Design review of the part built by this model. Coordinates are the model's own, in mm. Face numbers are marked on the shaded views. A direction names the side the tool comes from. Coordinates: 2 decimals unless noted, no trailing zeros. Loops run counter-clockwise (first coordinate to the right, second up) from the corner with the lowest first, then second, coordinate; pieces in that order, holes last. Notation, with made-up numbers: (38, 13.5) - (79, 13.5) arc R14 cw to (79, 37.5) - close; hole circle Ø10 at (57, -1). An arc over 180 degrees is marked (long way). Use one line per item in the form item = value. Start each with the question number.
(1) Add section D-D (x = -12). State the section outline as (y, z) points, plus the area to 3 significant figures.
(2) For L1, parallel to Y at x = -14.65, z = 0; L2, parallel to X at y = -7.25, z = -5; L3, parallel to Z at x = 39.5, y = -3.75, list the stretches that pass through material, from the lowest coordinate up.
(3) The part is to be moulded in two halves that separate along Z. For the marked faces 1, 2 and 3, say which applies: pulls with the +Z half, pulls with the -Z half, needs draft (parallel to the pull), parting line crosses it, or undercut.
(4) Tool access review of the marked faces 4, 5 and 6: name each direction out of +Z, -Z, +X, -X, +Y, -Y from which nothing blocks a thin tool from reaching the whole face with its end or side.
(5) Clearance check with flat-ended pins moving along their axes: pin 1 Ø3 at (x, y) = (12.5, -6) entering from -Z; pin 2 Ø8 at (x, z) = (37.5, 5.5) entering from +Y; pin 3 Ø1 at (y, z) = (-8, -1.5) entering from -X. State where each tip first meets the part, or that it passes through.
(6) Add section C-C (x = 0). State the section outline as (y, z) points.
(7) Add section A-A (y = 0). State the section outline as (x, z) points.
(8) Add section B-B (x = 24.5). State the section outline as (y, z) points, plus the area to 3 significant figures.
```python
from build123d import *

# Parameters (mm, degrees)
SKETCH_3_W               = 10
SKETCH_3_H               = 2
CUT_EXTRUDE_1_DEPTH      = 46.803930098
PATTERN_CIRCULAR_1_COUNT = 2
PATTERN_CIRCULAR_2_COUNT = 3


with BuildPart() as part:
    # Эскиз1 → Повернуть1 (revolve)
    with BuildSketch(Plane.XY, mode=Mode.PRIVATE) as revolve_1_sk:
        Polygon((-16, 2.55), (-16, 4.75), (-14.6, 4.75), (-14.6, 6.75), (-16, 6.75), (-16, 7.4), (-14.4, 9), (44, 9), (44, 4.5), (-13, 4.5), (-13, 2.55), align=None)
    revolve(revolve_1_sk.sketch.rotate(Axis((-16, 0, 0), (1, 0, 0)), 90), axis=Axis((-16, 0, 0), (1, 0, 0)))

    # Эскиз2 → Вырез-Повернуть1 (revolve, cut)
    with BuildSketch(Plane.XY, mode=Mode.PRIVATE) as cut_revolve_1_sk:
        Polygon((0, 0), (0, 9), (3.3, 9), (3.3, 5), (2.3, 5), (2.3, 0), align=None)
    revolve(cut_revolve_1_sk.sketch.rotate(Axis((0, 0, 0), (0, 1, 0)), 90), axis=Axis((0, 0, 0), (0, 1, 0)), mode=Mode.SUBTRACT)

    # Эскиз3 → Вырез-Вытянуть1 (cut, symmetric)
    with BuildSketch(Plane.XY):
        with Locations((27, 8)):
            Rectangle(SKETCH_3_W, SKETCH_3_H)
    cut_extrude_1 = extrude(amount=CUT_EXTRUDE_1_DEPTH, both=True, mode=Mode.SUBTRACT)

    # Эскиз5 → Отверстие обработанное метчиком M21 (revolve, cut)
    with BuildSketch(Plane(origin=(44, 6.5, 0), x_dir=(0, 0, -1), z_dir=(0, 1, 0))):
        Polygon((0, 0), (0, 8.480688495), (0.8, 8), (0.8, 0.3), (1.1, 0), align=None)
    hole_wizard_m21 = revolve(axis=Axis((50.35, 6.5, 0), (-1, 0, 0)), mode=Mode.SUBTRACT)

    # Круговой массив1: Вырез-Вытянуть1 ×2 about axis
    pattern_circular_1_axis = Axis((-41.040855915, 0, 0), (1, 0, 0))
    for i in range(1, PATTERN_CIRCULAR_1_COUNT):
        add(cut_extrude_1.rotate(pattern_circular_1_axis, i * 360 / PATTERN_CIRCULAR_1_COUNT), mode=Mode.SUBTRACT)

    # Круговой массив2: Отверстие обработанное метчиком M21 ×3 about axis
    pattern_circular_2_axis = Axis((0, 0, 0), (1, 0, 0))
    for i in range(1, PATTERN_CIRCULAR_2_COUNT):
        add(hole_wizard_m21.rotate(pattern_circular_2_axis, i * 360 / PATTERN_CIRCULAR_2_COUNT), mode=Mode.SUBTRACT)


solid = part.part
```
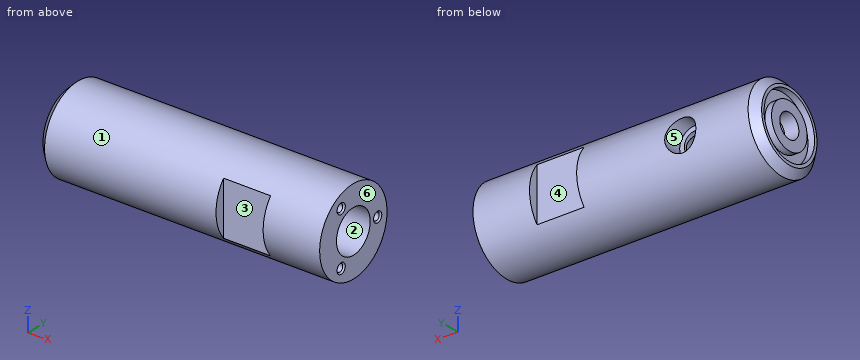
Computed values:
q1.outline = circle Ø18 at (0, 0); hole circle Ø9 at (0, 0)
q1.area = 191 mm^2
q2.L1 = -8.75 to -6.75, -4.75 to -2.55, 2.55 to 4.75, 6.75 to 8.75
q2.L2 = -14.59 to 22, 32 to 44
q2.L3 = -8.18 to -6.25, -5 to -2.49, 2.49 to 5, 6.25 to 8.18
q3.face_1 = parting line crosses it
q3.face_2 = undercut
q3.face_3 = needs draft
q4.face_4 = +Z, -Z, +Y
q4.face_5 = +Y
q4.face_6 = +Z, -Z, +X, +Y, -Y
q5.pin_1 = -7.79
q5.pin_2 = 8.87
q5.pin_3 = -15.76
q6.outline = (3.87, -2.3) arc R4.5 cw (long way) to (3.87, 2.3) - (5, 2.3) - (5, 3.3) - (8.37, 3.3) arc R9 ccw (long way) to (8.37, -3.3) - (5, -3.3) - (5, -2.3) - close
q7.outline = (-16, -7.4) - (-14.4, -9) - (44, -9) - (44, -4.5) - (-13, -4.5) - (-13, -2.55) - (-16, -2.55) - (-16, -4.75) - (-14.6, -4.75) - (-14.6, -6.75) - (-16, -6.75) - close; (-16, 2.55) - (-13, 2.55) - (-13, 4.5) - (44, 4.5) - (44, 9) - (-14.4, 9) - (-16, 7.4) - (-16, 6.75) - (-14.6, 6.75) - (-14.6, 4.75) - (-16, 4.75) - close
q8.outline = (-7, -5.66) arc R9 ccw to (7, -5.66) - (7, 5.66) arc R9 ccw to (-7, 5.66) - close; hole circle Ø9 at (0, 0)
q8.area = 160 mm^2
